Autodesk Inventor part; units mm, degrees
ref_plane "Work Plane1" through (29, 0, 0) normal (0, -1, 0) x (1, 0, 0)
ref_plane "YZ Plane" through (0, 0, 0) normal (1, 0, 0) x (0, 1, 0)
ref_plane "XZ Plane" through (0, 0, 0) normal (0, 1, 0) x (-1, 0, 0)
sketch "Sketch1" plane through (0, 0, 0) normal (0, 0, 1) x (1, 0, 0)
  line L0 (0.2879, 0) -> (7.9375, 0)
  line L1 (7.9375, 0) -> (7.9375, 2.413)
  line L2 (7.9375, 2.413) -> (2.0957, 2.413)
  line L3 (2.0957, 2.413) -> (0.0001, 2.413)
  line L4 (0.0001, 2.413) -> (0, 2.413)
  line L5 (0, 2.413) -> (0, 4.5847)
  line L6 (0, 4.5847) -> (-2.5654, 4.5847)
  line L7 (-2.5654, 4.5847) -> (-2.5654, 1.8624)
  line L8 (-2.5654, 1.8624) -> (-0.7874, 1.8624)
  line L9 (-0.7874, 1.8624) -> (0.2879, 0)
  line L10 (-4.666, 0) -> (10.0381, 0)
  line L11 (0, -0.9169) -> (0, 5.5016)
  line L12 (2.0957, 2.413) -> (0, 2.413) construction
  dimension "d1" = 5.8418
  dimension "d2" = 2.0956
  dimension "d3" = 2.5654
  dimension "d4" = 1.778
  dimension "d5" = 60
  dimension "d6" = 4.826
  dimension "d7" = 4.826
  dimension "d8" = 3.7248
  dimension "d9" = 9.1694
  dimension "d26" = 7.9375
revolve "Body" add sketch "Sketch1" angle 360 about axis through (0.2879, 0, 0) along (1, 0, 0) contours L9 L11 L3 L2 L1 L0 | L9 L8 L7 L6 L5 L11
sketch "Sketch2" plane through (-2.5654, 0, 0) normal (-1, 0, 0) x (0, 0, 1)
  circle A0 centre (0, 0) radius 1.8624
  line L0 (0, -6.4186) -> (0, 6.4186)
  line L1 (-6.4186, 0) -> (6.4186, 0)
  line L2 (1.8624, 0) -> (0.9312, -1.6129)
  line L3 (0.9312, -1.6129) -> (-0.9312, -1.6129)
  line L4 (-0.9312, -1.6129) -> (-1.8624, 0)
  line L5 (-1.8624, 0) -> (-0.9312, 1.6129)
  line L6 (-0.9312, 1.6129) -> (0.9312, 1.6129)
  line L7 (0.9312, 1.6129) -> (1.8624, 0)
  point P0 (0, 0)
extrude "Slot" add sketch "Sketch2" against normal up to next contours L7 A0 | A0 L2 | L6 L0 A0 | A0 L0 L3 | L0 L6 A0 | A0 L3 L0 | L4 A0 | A0 L5
fillet "Fillet1" radius 1.778 1 edges at (-2.5654, -4.5847, 0)
thread "Thread"
chamfer "Chamfer1" distance 0.6492 distance2 0.6492 1 edges at (7.9375, -2.413, 0) measured on face at (7.9375, -0.2686, 0.7084)
ref_plane "Work Plane1" through (29, 0, 0) normal (0, -1, 0) x (1, 0, 0)
fillet "Fillet2" radius 0.1 1 edges at (0.0001, -2.413, 0)
equation "\"d30\" = R"
equation "\"d17\" = RR"
equation "\"d13\" = GEL"
equation "\"d15\" = -0.5 * SPD + 0.5 * GD"
equation "\"d16\" = GUL"
equation "\"d1\" = GEL"
equation "\"d3\" = KOH"
equation "\"d4\" = INTI"
equation "\"d6\" = GD"
equation "\"d7\" = BDM"
equation "\"d8\" = 1.1547 * SW"
equation "\"d9\" = KOD"
equation "\"d26\" = NLG"
equation "\"GD\" = NND"
equation "\"NLG\" = 7.9375"
equation "\"GEL\" = 5.8418"
equation "\"KOD\" = 9.1694"
equation "\"KOH\" = 2.5654"
equation "\"INTI\" = 1.778"
equation "\"GAL\" = 2.0955"
equation "\"GUL\" = 0.64922"
equation "\"BDM\" = NND"
equation "\"SW\" = 3.2258"
equation "\"RR\" = 1.778"
equation "\"SPD\" = GD1"
equation "\"R\" = 0.1"
equation "\"KR\" = 5.4102"
equation "\"GD1\" = 3.52755"
equation "\"THREADDIA\" = 4.826"
equation "\"FAWI\" = 45deg"
equation "\"KOH1\" = 1.778"
equation "\"NND\" = 4.826"
equation "\"TOA\" = 30deg"
equation "\"E0\" = 1.155 * SW"
properties part number "Unbrako - 10 x 5/16" material "Steel, Mild"
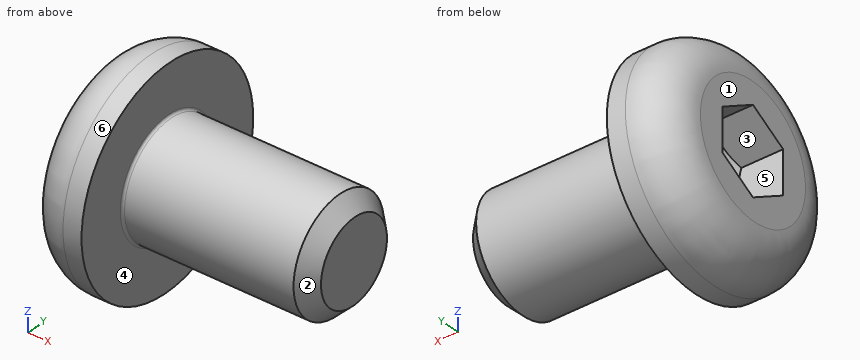
Geometry check sheet. Reference: the model listing, model coordinates, mm. Face numbers are marked on the shaded views. A direction names the side the tool comes from. Coordinates: 2 decimals unless noted, no trailing zeros. Order: outer loops, then holes, each group sorted by start corner. A loop starts at its lowest first (then second) coordinate and runs counter-clockwise, first axis right, second up. Notation, with made-up numbers: (1.25, 80.5) - (27.25, 80.5) arc R13 ccw to (27.25, 99.5) - close; hole circle Ø11 at (88, 65.5). An arc over 180 degrees is marked (long way). Answer in a Markdown table with one row per item. Add a question column.
1. Section check B-B (x = 5). Enter the section's corners in (y, z).
2. Section check A-A (x = -2). Enter the section's corners in (y, z).
3. Draft check along Y on the marked faces 1, 2 and 3. Enter one of: +Y half, -Y half, draft (parallel to the pull), parting line (faces both ways), or undercut.
4. Material ranges on L1, parallel to X at y = 0.25, z = 2.5; L2, parallel to Z at x = -0.25, y = 0.5; L3, parallel to Y at x = 7, z = 0.75, recorded low to high. Write a range as [from, to].
5. Gauge pin test, flat ends, axial feed: pin 1 Ø2 at (x, z) = (-2, 0) entering from -Y; pin 2 Ø4 at (x, z) = (3.5, -0.5) entering from -Y; pin 3 Ø5 at (x, z) = (4.5, 0) entering from +Y. Record the tip position at first contact, or that the pin passes through.
6. Access from +Z, -Z, +X, -X, +Y, -Y to the whole of each face (thin tool, end or side, straight path). Record for the marked faces 4, 5 and 6.
Data:
| question | item | result |
|---|---|---|
| 1 | outline | circle Ø4.83 at (0, 0) |
| 2 | outline | circle Ø8.21 at (0, 0); hole (-1.61, -0.93) - (0, -1.86) - (1.61, -0.93) - (1.61, 0.93) - (0, 1.86) - (-1.61, 0.93) - close |
| 3 | face 1 | draft |
| 3 | face 2 | parting line |
| 3 | face 3 | undercut |
| 4 | L1 | x = [-2.57, 0] |
| 4 | L2 | z = [-4.56, -0.79], [0.79, 4.56] |
| 4 | L3 | y = [-2.29, 2.29] |
| 5 | pin 1 | stops at y = -4.57 |
| 5 | pin 2 | stops at y = -2.41 |
| 5 | pin 3 | stops at y = 2.41 |
| 6 | face 4 | +X |
| 6 | face 5 | -X |
| 6 | face 6 | +X, -X |
